Source: CAD feature listing. Evaluate the final solid. Frame: model axes, mm. A direction names the side the tool comes from. Coordinates: 2 decimals unless noted, no trailing zeros. Order: outer loops, then holes, each group sorted by start corner. A loop starts at its lowest first (then second) coordinate and runs counter-clockwise, first axis right, second up.
```python
from build123d import *

# Parameters (mm, degrees)
F0_W     = 38.1
F0_H     = 25.4
F1_DEPTH = 2.54
F2_W     = 5.08
F2_H     = 5.08
F3_DEPTH = 15.24


with BuildPart() as f1:
    # F0 (on Front) → F1 (new body)
    with BuildSketch(Plane.XZ):
        with Locations((19.05, -12.7)):
            Rectangle(F0_W, F0_H)
    extrude(amount=F1_DEPTH)

    # F2 (on face) → F3 (join)
    with BuildSketch(Plane(origin=(0, 0, 0), x_dir=(-1, 0, 0), z_dir=(0, 1, 0))):
        with Locations((-35.56, -2.54)):
            Rectangle(F2_W, F2_H)
        with Locations((-35.56, -22.86)):
            Rectangle(F2_W, F2_H)
        with Locations((-2.54, -2.54)):
            Rectangle(F2_W, F2_H)
        with Locations((-2.54, -22.86)):
            Rectangle(F2_W, F2_H)
    extrude(amount=F3_DEPTH)


solid = f1.part
```
1. Section query D-D, the plane x = 9. Output: boundary loops of the cut face in (y, z), plus the area to 3 significant figures.
2. Section query B-B, the plane x = 4. Output: boundary loops of the cut face in (y, z).
3. Access query for faces 5 (the flat face through (36, 8, -5.08)), 6 (the flat face through (33.02, 8, -3)), 7 (the flat face through (19, -0.2, -25.4)). Directions: +Z, -Z, +X, -X, +Y, -Y. A direction counts if a zero-diameter tool reaches every point of the face in a straight line with its end or side. Return the directions, or none.
4. Draft query along X for faces 1 (the flat face through (0, -1, -13)), 2 (the flat face through (36, 15.24, -3)), 3 (the flat face through (5.08, 8, -3)), 4 (the flat face through (19, 0, -13)). Return one class per face: +X half, -X half, draft (parallel to the pull), parting line (faces both ways), or undercut.
5. Material intervals for line 1 along Z through (x, y) = (36, 13.25); line 2 along X through (y, z) = (12.75, -3.75); line 3 along Y through (x, z) = (26.5, -13), sorted ascending.
6. Contact query for flat-ended pins moving along their axis: P1, Ø2.5, axis at y = 4.5, z = -23.5, coming from the -X side; P2, Ø3, axis at x = 10, z = -6, coming from the +Y side. Output: stop coordinate, or through.
7. Section query C-C, the plane z = -23.5. Output: boundary loops of the cut face in (x, y), plus the area to 3 significant figures.
8. Section query A-A, the plane y = 12. Output: boundary loops of the cut face in (x, z).
Answer key:
1. outline: (-2.54, -25.4) - (0, -25.4) - (0, 0) - (-2.54, 0) - close
1. area: 64.5 mm2
2. outline: (-2.54, -25.4) - (15.24, -25.4) - (15.24, -20.32) - (0, -20.32) - (0, -5.08) - (15.24, -5.08) - (15.24, 0) - (-2.54, 0) - close
3. face 5: +X, -X, +Y
3. face 6: +Z, -Z, +Y
3. face 7: -Z, +X, -X, +Y, -Y
4. face 1: -X half
4. face 2: draft
4. face 3: undercut
4. face 4: undercut
5. line 1: z = -25.4 to -20.32, -5.08 to 0
5. line 2: x = 0 to 5.08, 33.02 to 38.1
5. line 3: y = -2.54 to 0
6. P1: stops at x = 0
6. P2: stops at y = 0
7. outline: (0, -2.54) - (38.1, -2.54) - (38.1, 15.24) - (33.02, 15.24) - (33.02, 0) - (5.08, 0) - (5.08, 15.24) - (0, 15.24) - close
7. area: 252 mm2
8. outline: (0, -25.4) - (5.08, -25.4) - (5.08, -20.32) - (0, -20.32) - close; (0, -5.08) - (5.08, -5.08) - (5.08, 0) - (0, 0) - close; (33.02, -25.4) - (38.1, -25.4) - (38.1, -20.32) - (33.02, -20.32) - close; (33.02, -5.08) - (38.1, -5.08) - (38.1, 0) - (33.02, 0) - close
